from build123d import *

# Parameters (mm, degrees)
SKETCH_1_R             = 8.5
EXTRUDE_1_DEPTH        = 20
SKETCH_2_R             = 7.5
EXTRUDE_2_DEPTH        = 5
SKETCH_3_R             = 8.5
SKETCH_3_R_2           = 8
CUT_EXTRUDE_1_DEPTH    = 1
SKETCH_5_R             = 13.5
EXTRUDE_3_DEPTH        = 4
SKETCH_7_R             = 7.5
EXTRUDE_4_DEPTH        = 6
SKETCH_9_R             = 5
CUT_EXTRUDE_3_DEPTH    = 36
CHAMFER_2_SIZE         = 0.5
CUT_EXTRUDE_4_DEPTH    = 7
SKETCH_12_W            = 4
SKETCH_12_H            = 7
CUT_EXTRUDE_5_DEPTH    = 18.1
CHAMFER_3_SIZE         = 0.5
CHAMFER_4_SIZE         = 1
FILLET_1_R             = 0.2
HOLE_WIZARD_M3_1_D     = 2.5
HOLE_WIZARD_M3_1_DEPTH = 4


with BuildPart() as part:
    # 草图1 → 凸台-拉伸1 (new body)
    with BuildSketch(Plane.XY):
        Circle(SKETCH_1_R)
    extrude(amount=EXTRUDE_1_DEPTH)

    # 草图2 → 凸台-拉伸2 (add)
    with BuildSketch(Plane.XY.offset(20)):
        Circle(SKETCH_2_R)
    extrude(amount=EXTRUDE_2_DEPTH)

    # 草图3 → 切除-拉伸1 (cut)
    with BuildSketch(Plane.XY.offset(8)):
        Circle(SKETCH_3_R)
        Circle(SKETCH_3_R_2, mode=Mode.SUBTRACT)
    extrude(amount=CUT_EXTRUDE_1_DEPTH, mode=Mode.SUBTRACT)

    # 草图5 → 凸台-拉伸3 (add)
    with BuildSketch(Plane(origin=(0, 0, 0), x_dir=(-1, 0, 0), z_dir=(0, 0, -1))):
        Circle(SKETCH_5_R)
    extrude(amount=EXTRUDE_3_DEPTH)

    # 草图7 → 凸台-拉伸4 (add)
    with BuildSketch(Plane(origin=(0, 0, -4), x_dir=(-1, 0, 0), z_dir=(0, 0, -1))):
        Circle(SKETCH_7_R)
    extrude(amount=EXTRUDE_4_DEPTH)

    # 草图9 → 切除-拉伸3 (cut, through all)
    with BuildSketch(Plane(origin=(0, 0, -10), x_dir=(-1, 0, 0), z_dir=(0, 0, -1))):
        Circle(SKETCH_9_R)
    extrude(amount=-CUT_EXTRUDE_3_DEPTH, mode=Mode.SUBTRACT)

    # 倒角2
    chamfer_2_edges = [part.edges().sort_by_distance(p)[0] for p in [
        (7.5, 0, -10),
    ]]
    chamfer(chamfer_2_edges, length=CHAMFER_2_SIZE)

    # 草图10 → 切除-拉伸4 (cut)
    with BuildSketch(Plane.XY.offset(18)):
        with BuildLine():
            Line((-7.7, 3.6), (7.7, 3.6))
            ThreePointArc((7.7, 3.6), (0, 8.5), (-7.7, 3.6))
        make_face()
        with BuildLine():
            Line((-6.020797289, -6), (6.020797289, -6))
            ThreePointArc((6.020797289, -6), (0, -8.5), (-6.020797289, -6))
        make_face()
    extrude(amount=-CUT_EXTRUDE_4_DEPTH, mode=Mode.SUBTRACT)

    # 草图12 → 切除-拉伸5 (cut, through all)
    with BuildSketch(Plane(origin=(0, 3.6, 0), x_dir=(1, 0, 0), z_dir=(0, 1, 0))):
        with Locations((-8.5, -14.5)):
            Rectangle(SKETCH_12_W, SKETCH_12_H)
        with Locations((8.5, -14.5)):
            Rectangle(SKETCH_12_W, SKETCH_12_H)
    extrude(amount=-CUT_EXTRUDE_5_DEPTH, mode=Mode.SUBTRACT)

    # 倒角3
    chamfer_3_edges = [part.edges().sort_by_distance(p)[0] for p in [
        (5, 0, 25),
    ]]
    chamfer(chamfer_3_edges, length=CHAMFER_3_SIZE)

    # 倒角4
    chamfer_4_edges = [part.edges().sort_by_distance(p)[0] for p in [
        (-6.5, 3.6, 14.5),
        (6.5, 3.6, 14.5),
    ]]
    chamfer(chamfer_4_edges, length=CHAMFER_4_SIZE)

    # 圆角1
    fillet_1_edges = [part.edges().sort_by_distance(p)[0] for p in [
        (3.469870315, 3.6, 14.5),
        (-3.469870315, 3.6, 14.5),
    ]]
    fillet(fillet_1_edges, radius=FILLET_1_R)

    # M3 螺纹孔1
    with Locations(Plane(origin=(0, 0, -4), x_dir=(-1, 0, 0), z_dir=(0, 0, -1))):
        with Locations((-10.5, 0), (0, 10.5), (10.5, 0), (0, -10.5)):
            Hole(HOLE_WIZARD_M3_1_D / 2, depth=HOLE_WIZARD_M3_1_DEPTH)


solid = part.part
Input: part model. Units: mm. Frame: model coordinates. A direction names the side the tool comes from. Give positions to 0.01 mm unless a question says otherwise; leave off trailing zeros. Write each loop counter-clockwise with the first axis right and the second up, starting at its lowest first coordinate (ties: lowest second). Pieces come first, ordered by that corner, then holes. Notation, with made-up numbers: M 53.5,54 L 68.5,54 A17 ccw 68.5,72 Z; hole C 6,19 d2. An arc over 180 degrees is marked long. Write item = value, one per line. Start each with the question number.
1) First-contact query: pin 1 Ø0.8 at (x, y) = (0.5, -7.5) entering from -Z; pin 2 Ø1.7 at (x, z) = (5, 15) entering from +Y; pin 3 Ø8.5 at (x, y) = (0, -0.5) entering from +Z; pin 4 Ø5 at (y, z) = (-3.5, 12) entering from +X. Flat tips, straight axial feed; report the tip coordinate or a pass-through.
2) Cut plane C-C on x = -10.5. Return the cut outline in (y, z), then the cut area to 3 significant figures.
3) Cut plane B-B on y = 11.25. Return the cut outline in (x, z).
4) Cut plane D-D on x = -1.75. Count the separate pieces of the cut face and the enclosed holes in it, then the cut area to 3 significant figures.
5) Draft query along X for faces 4 (the cylindrical face through (-0.16, 11.74, -1.97)), 5 (the flat face through (6, 3.1, 14.5)), 6 (the cylindrical face through (-2.307, -4.436, 7.009)), 7 (the flat face through (-5, 3.6, 15)). Return one class per face: +X half, -X half, draft (parallel to the pull), parting line (faces both ways), or undercut.
6) Cut plane A-A on z = -2.5. Return the cut outline in (x, y), then the cut area to 3 significant figures.
7) Reachability of faces 1 (the flat face through (6.5, -1, 15)), 2 (the cylindrical face through (7.493, 0.33, -6.712)), 3 (the flat face through (0.6, 5.2, 11)) from +Z, -Z, +X, -X, +Y, -Y: full face, straight path, thin tool, end or side. Return the list, or none.
8) Material intervals for line 1 along Y through (x, z) = (0, -2.45); line 2 along Z through (x, y) = (-6, 11); line 3 along Y through (x, z) = (-10.5, -3.05), sorted ascending. Write a range as [from, to].
Solved:
q1.pin_1 = -9.88
q1.pin_2 = 3.6
q1.pin_3 = through
q1.pin_4 = 8.41
q2.outline = M -8.49,-4 L -1.25,-4 L -1.25,0 L -8.49,0 Z; M 1.25,-4 L 8.49,-4 L 8.49,0 L 1.25,0 Z
q2.area = 57.9 mm2
q3.outline = M -7.46,-4 L -1,-4 L -1,0 L -7.46,0 Z; M 1,-4 L 7.46,-4 L 7.46,0 L 1,0 Z
q4.separate_pieces = 3
q4.enclosed_holes = 0
q4.area = 229 mm2
q5.face_4 = undercut
q5.face_5 = +X half
q5.face_6 = undercut
q5.face_7 = draft
q6.outline = C 0,0 d27; hole C -10.5,0 d2.5; hole C 0,0 d10; hole C 0,-10.5 d2.5; hole C 0,10.5 d2.5; hole C 10.5,0 d2.5
q6.area = 474 mm2
q7.face_1 = +X, +Y, -Y
q7.face_2 = -Z
q7.face_3 = +Y
q8.line_1 = [-13.5, -11.75], [-9.25, -5], [5, 9.25], [11.75, 13.5]
q8.line_2 = [-4, 0]
q8.line_3 = [-8.49, -1.25], [1.25, 8.49]
